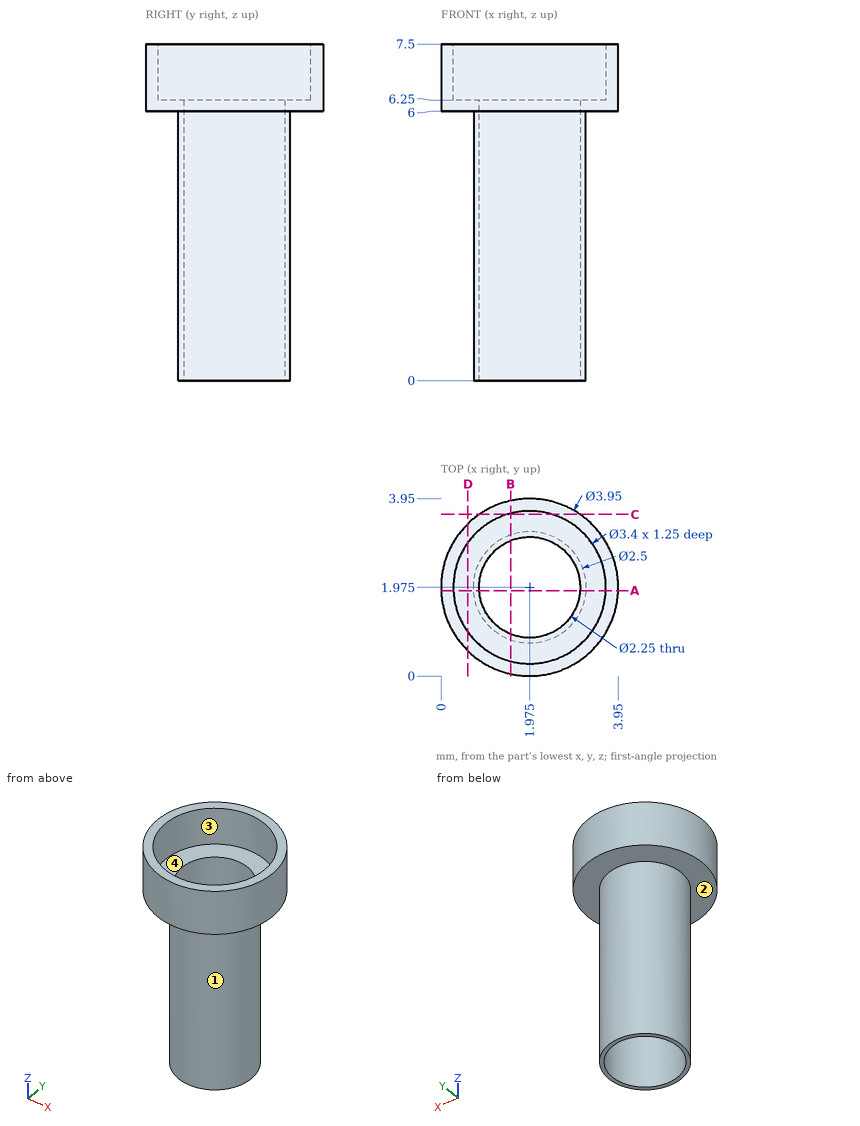
Geometry check sheet. Reference: drawing and pictorial views, mm from the part's lowest x, y, z. Coordinates: 2 decimals unless noted, no trailing zeros. Order: outer loops, then holes, each group sorted by start corner. A loop starts at its lowest first (then second) coordinate and runs counter-clockwise, first axis right, second up. Notation, with made-up numbers: M -21.75,-32 L 28.25,-32 A21 ccw 28.25,-7 Z; hole C 81,45 d11. An arc over 180 degrees is marked long. Return JSON: item names as keys, results as strings.
1) Thickness scan on L1, parallel to Y at x = 1.95, z = 6.75; L2, parallel to Y at x = 1.2, z = 2; L3, parallel to Z at x = 3, y = 2.6. Record the ranges inside material, lowest first. Write a range as [from, to].
Answer list:
{"L1": "[0, 0.28], [3.67, 3.95]", "L2": "[0.99, 1.16], [2.79, 2.96]", "L3": "[0, 6.25]"}
2) Cross-section at A-A, the plane y = 1.9. Record the boundary of the cut face in (x, z), and give its area (3 significant figures).
Answer list:
{"outline": "M 0,6 L 0.73,6 L 0.73,0 L 0.85,0 L 0.85,6.25 L 0.28,6.25 L 0.28,7.5 L 0,7.5 Z; M 3.1,0 L 3.22,0 L 3.22,6 L 3.95,6 L 3.95,7.5 L 3.67,7.5 L 3.67,6.25 L 3.1,6.25 Z", "area": "2.62 mm2"}
3) Cross-section at C-C, the plane y = 3.6. Record the boundary of the cut face in (x, z).
Answer list:
{"outline": "M 0.85,6 L 3.1,6 L 3.1,7.5 L 2.47,7.5 L 2.47,6.25 L 1.48,6.25 L 1.48,7.5 L 0.85,7.5 Z"}
4) Cross-section at B-B, the plane x = 1.55. Record the boundary of the cut face in (y, z).
Answer list:
{"outline": "M 0.05,6 L 0.8,6 L 0.8,0 L 0.93,0 L 0.93,6.25 L 0.33,6.25 L 0.33,7.5 L 0.05,7.5 Z; M 3.02,0 L 3.15,0 L 3.15,6 L 3.9,6 L 3.9,7.5 L 3.62,7.5 L 3.62,6.25 L 3.02,6.25 Z"}
5) Cross-section at D-D, the plane x = 0.6. Record the boundary of the cut face in (y, z).
Answer list:
{"outline": "M 0.56,6 L 3.39,6 L 3.39,7.5 L 2.97,7.5 L 2.97,6.25 L 0.98,6.25 L 0.98,7.5 L 0.56,7.5 Z"}
6) Release check for a two-part mould opening along Y. For the marked faces 1, 2, 3 and 4 record: +Y half, -Y half, draft (parallel to the pull), parting line (faces both ways), or undercut.
Answer list:
{"face 1": "parting line", "face 2": "draft", "face 3": "undercut", "face 4": "undercut"}
7) Gauge pin test, flat ends, axial feed: pin 1 (1.5 mm diameter, centred on y = 2.5, z = 1.5, fed in from +X) (3 decimals); pin 2 (1.2 mm diameter, centred on x = 1.5, y = 2.5, fed in from -Z); pin 3 (1.8 mm diameter, centred on x = 1.975, y = 1.975, fed in from -Z); pin 4 (2 mm diameter, centred on x = 0.5, z = 4, fed in from +Y). Record the tip position at first contact, or that the pin passes through.
Answer list:
{"pin 1": "x = 3.225", "pin 2": "z = 0", "pin 3": "through", "pin 4": "y = 3.13"}
